The model under review builds one solid part; all positions refer to its coordinate system, in mm. A direction names the side the tool comes from. Round coordinates to 2 decimals unless told otherwise and drop trailing zeros. Order: outer loops, then holes, each group sorted by start corner. A loop starts at its lowest first (then second) coordinate and runs counter-clockwise, first axis right, second up. Notation, with made-up numbers: M 13,28 L 18,28 A13 ccw 18,37 Z; hole C 85.25,83.25 d4. An arc over 180 degrees is marked long. Answer as CSV lines item,"result". Start each with the question number.
Autodesk Inventor part; units mm, degrees
ref_plane "YZ Plane" through (0, 0, 0) normal (1, 0, 0) x (0, 1, 0)
ref_plane "XZ Plane" through (0, 0, 0) normal (0, 1, 0) x (-1, 0, 0)
ref_plane "XY Plane" through (0, 0, 0) normal (0, 0, 1) x (1, 0, 0)
sketch "Sketch1" plane through (0, 0, 0) normal (0, 0, 1) x (1, 0, 0)
  line L0 (-20, 16.5858) -> (-16.5858, 20)
  line L1 (-20, -16.5858) -> (-20, 16.5858)
  line L2 (-16.5858, -20) -> (-20, -16.5858)
  line L3 (16.5858, -20) -> (-16.5858, -20)
  line L4 (20, -16.5858) -> (16.5858, -20)
  line L5 (20, 16.5858) -> (20, -16.5858)
  line L6 (16.5858, 20) -> (20, 16.5858)
  line L7 (-16.5858, 20) -> (16.5858, 20)
  circle A0 centre (15.5, -15.5) radius 1.5
  circle A1 centre (-15.5, 15.5) radius 1.5
  circle A2 centre (-15.5, -15.5) radius 1.5
  circle A3 centre (15.5, 15.5) radius 1.5
  circle A4 centre (0, 0) radius 11
  line L8 (-20, 0) -> (-30, 0) construction
  line L9 (-20, 0) -> (-20, -30)
  line L10 (-20, -30) -> (-30, -30)
  line L11 (-30, -30) -> (-30, 30)
  line L12 (-30, 30) -> (-20, 30)
  line L13 (-20, 30) -> (-20, -30)
  line L14 (-15.5, -17) -> (-20, -17)
  line L15 (-20, 17) -> (-15.5, 17)
  line L16 (0, 0) -> (100, 0.0668) construction
  circle A5 centre (0, 0) radius 3.8 construction
  circle A6 centre (0, 0) radius 4 construction
  line L17 (0, 0) -> (100, 0.0668) construction
  line L18 (0.0027, -4) -> (100.0026, -3.9332)
  line L19 (99.9973, 4.0668) -> (-0.0027, 4)
  arc A7 (-0.0027, 4) -> (0.0027, -4) centre (0, 0) ccw
  arc A8 (100.0026, -3.9332) -> (99.9973, 4.0668) centre (100, 0.0668) ccw
  line L20 (15.5, -15.5) -> (0, -15.5) construction
  line L21 (15.5, -15.5) -> (115.5, -15.5) construction
  line L22 (15.5, 15.5) -> (115.5, 15.5) construction
  line L23 (115.5, 15.5) -> (115.5, -15.5) construction
  circle A9 centre (-15.5, -15.5) radius 1.7 construction
  circle A10 centre (-15.5, 15.5) radius 1.7 construction
  line L24 (-15.5, 15.5) -> (115.5, 15.5) construction
  line L25 (-15.5, 17.2) -> (115.5, 17.2)
  line L26 (115.5, 13.8) -> (-15.5, 13.8)
  arc A11 (-15.5, 17.2) -> (-15.5, 13.8) centre (-15.5, 15.5) ccw
  arc A12 (115.5, 13.8) -> (115.5, 17.2) centre (115.5, 15.5) ccw
  line L27 (-15.5, -15.5) -> (115.5, -15.5) construction
  line L28 (-15.5, -13.8) -> (115.5, -13.8)
  line L29 (115.5, -17.2) -> (-15.5, -17.2)
  arc A13 (-15.5, -13.8) -> (-15.5, -17.2) centre (-15.5, -15.5) ccw
  arc A14 (115.5, -17.2) -> (115.5, -13.8) centre (115.5, -15.5) ccw
  line L30 (117.2, 15.5) -> (122.2, 15.5) construction
  line L31 (-20, 30) -> (122.2, 30)
  line L32 (122.2, 30) -> (122.2, -30)
  line L33 (122.2, -30) -> (-20, -30)
  point P0 (50, 0.0334)
  point P1 (50, 15.5)
  point P2 (50, -15.5)
  point P3 (-19.5858, 17)
  point P4 (19.3858, 17.2)
  point P5 (20, 13.8)
  point P6 (20, 4.0134)
  point P7 (20, -3.9866)
  point P8 (20, -13.8)
  point P9 (19.3858, -17.2)
  point P10 (-19.5858, -17)
  point P11 (-16.3, 17)
  dimension "d0" = 10
  dimension "d1" = 30
  dimension "d2" = 10
  dimension "d3" = 60
  dimension "d6" = 100
  dimension "d7" = 0.2
  dimension "d8" = 100
  dimension "d9" = 0.2
  dimension "d10" = 0.2
  dimension "d11" = 5
extrude "Extrusion1" add sketch "Sketch1" along normal blind 3 contours L0 L15 A11 L26 L5 L19 A4 L18 L28 A13 L14 L2 L1 | L1 L9 L10 L11 L12 L13 | L15 L13 L31 L32 L33 L9 L14 L2 L3 L4 L29 A14 L28 L5 L18 A8 L19 L26 A12 L25 L6 L7 L0 | L0 L7 L6 L25 A11 L15 | L14 A13 L29 L4 L3 L2 | L19 A7 L18 A4 picked at (6.4115, 4.7804)
sketch "Sketch2" plane through (-30, -30, 0) normal (-1, 0, 0) x (0, 0, 1)
  point P0 (0, 30)
sketch "Sketch3" plane through (-30, -30, 0) normal (-1, 0, 0) x (0, 0, 1)
  line L0 (0, 60) -> (0, 0)
  line L1 (0, 0) -> (3, 0)
  line L2 (3, 60) -> (3, 0)
  line L3 (0, 60) -> (3, 60)
  line L4 (8, -5) -> (-5, -5)
  line L5 (-5, -5) -> (-5, 65)
  line L6 (-5, 65) -> (8, 65)
  line L7 (8, 65) -> (8, -5)
  line L8 (0, 47.2) -> (0, 43.8)
  line L9 (-2.7217, 45.5) -> (3, 45.5)
  circle A0 centre (0.1391, 45.5) radius 1.5
  point P0 (0, 30)
  point P1 (-1.5323, 14.5)
  dimension "d15" = 5
  dimension "d16" = 3
sketch "Sketch4" plane through (0, 0, 0) normal (0, 0, -1) x (-1, 0, 0)
  line L0 (30, 30) -> (30, -30)
  line L1 (-122.2, 30) -> (30, 30)
  line L2 (-122.2, -30) -> (-122.2, 30)
  line L3 (30, -30) -> (-122.2, -30)
  line L4 (20, -16.5858) -> (19.5858, -17)
  line L5 (20, -17) -> (20, -16.5858)
  line L6 (19.5858, -17) -> (20, -17)
  arc A0 (15.5, 13.8) -> (15.5, 17.2) centre (15.5, 15.5) ccw
  line L7 (-115.5, 13.8) -> (15.5, 13.8)
  arc A1 (-115.5, 17.2) -> (-115.5, 13.8) centre (-115.5, 15.5) ccw
  line L8 (15.5, 17.2) -> (-115.5, 17.2)
  line L9 (-100.0026, -3.9332) -> (-0.0027, -4)
  arc A2 (-99.9973, 4.0668) -> (-100.0026, -3.9332) centre (-100, 0.0668) ccw
  line L10 (0.0027, 4) -> (-99.9973, 4.0668)
  arc A3 (-0.0027, -4) -> (0.0027, 4) centre (0, 0) ccw
  line L11 (15.5, -13.8) -> (-115.5, -13.8)
  arc A4 (15.5, -17.2) -> (15.5, -13.8) centre (15.5, -15.5) ccw
  line L12 (-115.5, -17.2) -> (15.5, -17.2)
  arc A5 (-115.5, -13.8) -> (-115.5, -17.2) centre (-115.5, -15.5) ccw
  line L13 (19.5858, 17) -> (20, 16.5858)
  line L14 (20, 17) -> (19.5858, 17)
  line L15 (20, 16.5858) -> (20, 17)
  line L16 (0, 0) -> (-100, 0.0668) construction
  line L17 (0.0075, 11.2) -> (-99.9925, 11.2668)
  line L18 (-100.0075, -11.1332) -> (-0.0075, -11.2)
  arc A6 (-0.0075, -11.2) -> (0.0075, 11.2) centre (0, 0) ccw
  arc A7 (-99.9925, 11.2668) -> (-100.0075, -11.1332) centre (-100, 0.0668) ccw
  point P0 (0, 0)
  point P1 (-50, 0.0334)
  dimension "d17" = 22.4
extrude "Extrusion2" cut sketch "Sketch4" against normal blind 2.2 contours A6 L18 A7 L17
properties part number "CombineTestHorizontal"
Item 1: Consider section C-C (y = 0.5). State the section outline as (x, z) points.
Item 2: Consider section B-B (z = 0.55). State the section outline as (x, y) points, and give its area (3 significant figures).
Item 3: The part is to be moulded in two halves that separate along X. For faces 4 (the flat face through (51, -17.2, 1)), 5 (the flat face through (51, -5, 2.2)), 6 (the flat face through (45, -13, 0)), 7 (the flat face through (-30, 0, 1)), say which applies: +X half, -X half, draft (parallel to the pull), parting line (faces both ways), or undercut.
Item 4: Consider section D-D (y = 9). State the section outline as (x, z) points.
Item 5: Tool access review of faces 1 (the cylindrical face through (117.2, -15.5, 1.5)), 2 (the flat face through (45, 7, 3)), 3 (the cylindrical face through (111.197, 0.321, 1.085)): name each direction out of +Z, -Z, +X, -X, +Y, -Y from which nothing blocks a thin tool from reaching the whole face with its end or side.
Item 6: Wall thickness on probe 1 along Y at (x, z) = (59.5, 1.15); probe 2 along Y at (x, z) = (64.5, 2.8); probe 3 along X at (y, z) = (-15.5, 2.5): over which ranges is each line inside the solid? List them lowest first. Write a range as [from, to].
Item 7: For pin 1 (4 mm diameter, centred on x = 82, y = 8.5, fed in from -Z), flat-tipped, find the tip position at first contact; note if it passes through.
Item 8: Consider section A-A (x = 86). State the section outline as (y, z) points, and give its area (3 significant figures).
Reported:
1,outline,"M -30,0 L -11.19,0 L -11.19,2.2 L -3.97,2.2 L -3.97,3 L -30,3 Z; M 103.98,2.2 L 111.19,2.2 L 111.19,0 L 122.2,0 L 122.2,3 L 103.98,3 Z"
2,outline,"M -30,-30 L 122.2,-30 L 122.2,30 L -30,30 Z; hole M -20,-17 L -19.59,-17 L -20,-16.59 Z; hole M -20,16.59 L -19.59,17 L -20,17 Z; hole M -15.5,-17.2 L 115.5,-17.2 A1.7 ccw 115.5,-13.8 L -15.5,-13.8 A1.7 ccw Z; hole M -15.5,13.8 L 115.5,13.8 A1.7 ccw 115.5,17.2 L -15.5,17.2 A1.7 ccw Z; hole M -0.01,11.2 A11.2 ccw 0.01,-11.2 L 100.01,-11.13 A11.2 ccw 99.99,11.27 Z"
2,area,"5,590 mm²"
3,face 4,"undercut"
3,face 5,"undercut"
3,face 6,"draft"
3,face 7,"-X half"
4,outline,"M -30,0 L -6.67,0 L -6.67,2.2 L 106.76,2.2 L 106.76,0 L 122.2,0 L 122.2,3 L -30,3 Z"
5,face 1,"+Z, -Z"
5,face 2,"+Z, +X, -X, +Y, -Y"
5,face 3,"-Z"
6,probe 1,"y = [-30, -17.2], [-13.8, -11.16], [11.24, 13.8], [17.2, 30]"
6,probe 2,"y = [-30, -17.2], [-13.8, -3.96], [4.04, 13.8], [17.2, 30]"
6,probe 3,"x = [-30, -17.2], [117.2, 122.2]"
7,pin 1,"stops at z = 2.2"
8,outline,"M -30,0 L -17.2,0 L -17.2,3 L -30,3 Z; M -13.8,0 L -11.14,0 L -11.14,2.2 L -3.94,2.2 L -3.94,3 L -13.8,3 Z; M 4.06,2.2 L 11.26,2.2 L 11.26,0 L 13.8,0 L 13.8,3 L 4.06,3 Z; M 17.2,0 L 30,0 L 30,3 L 17.2,3 Z"
8,area,"104 mm²"
